Autodesk Inventor part; units mm, degrees
ref_plane "Work Plane1" through (0, 0, 7.82) normal (0, 0, 1) x (1, 0, 0)
ref_plane "Work Plane2" through (0, 0, 11.74) normal (0, 0, 1) x (1, 0, 0)
ref_plane "Work Plane3" through (0, 0, 14) normal (0, 0, 1) x (1, 0, 0)
sketch "Base" plane through (0, 0, 0) normal (0, 0, 1) x (1, 0, 0)
  line L0 (-20.125, 20.125) -> (20.125, 20.125)
  line L1 (20.125, 20.125) -> (20.125, -20.125)
  line L2 (20.125, -20.125) -> (-20.125, -20.125)
  line L3 (-20.125, -20.125) -> (-20.125, 20.125)
  line L4 (-15.74, 20.125) -> (-20.125, 15.74)
  line L5 (15.74, 20.125) -> (20.125, 15.74)
  line L6 (-17.02, 17.02) -> (17.02, 17.02) construction
  line L7 (17.02, 17.02) -> (17.02, -17.02) construction
  line L8 (17.02, -17.02) -> (-17.02, -17.02) construction
  line L9 (-17.02, -17.02) -> (-17.02, 17.02) construction
  line L10 (-17.02, 17.02) -> (17.02, -17.02) construction
  line L11 (17.02, 17.02) -> (-17.02, -17.02) construction
  circle A0 centre (0, 0) radius 8.4
  circle A1 centre (17.02, 17.02) radius 1.05
  circle A2 centre (-17.02, 17.02) radius 1.05
  circle A3 centre (-17.02, -17.02) radius 1.05
  circle A4 centre (17.02, -17.02) radius 1.05
  line L12 (-20.125, -15.74) -> (-15.74, -20.125)
  line L13 (20.125, -15.74) -> (15.74, -20.125)
  point P0 (0, 0)
  point P1 (0, 0)
  dimension "d0" = 40.25
  dimension "d1" = 40.25
  dimension "d2" = 135
  dimension "d3" = 135
  dimension "d4" = 31.48
  dimension "d5" = 34.04
  dimension "d6" = 3.105
  dimension "d7" = 3.105
  dimension "d8" = 3.105
  dimension "d9" = 3.105
  dimension "d10" = 16.8
  dimension "d11" = 2.1
  dimension "d12" = 135
  dimension "d13" = 135
  dimension "d14" = 31.48
  dimension "d15" = 34.04
  dimension "d16" = 31.48
extrude "BaseFeature" add sketch "Base" along normal blind 1.5 contours L0 L5 L1 L13 L2 L12 L3 L4 | A0
extrude "CameraFeature" add sketch "Base" along normal blind 16 contours A0
sketch "Sketch2" plane through (0, 0, 16) normal (0, 0, 1) x (1, 0, 0)
  circle A0 centre (0, 0) radius 8.4
  circle A1 centre (0, 0) radius 4
  point P0 (0, 0)
  dimension "d28" = 8
extrude "Extrusion3" cut sketch "Sketch2" against normal blind 7.62 contours A1
sketch "Sketch4" plane through (0, 0, 1.5) normal (0, 0, 1) x (1, 0, 0)
  circle A0 centre (0, 0) radius 4
  circle A1 centre (0, 0) radius 8.4
  line L0 (-8.4, -8.4) -> (8.4, -8.4)
  line L1 (8.4, -8.4) -> (8.4, 8.4)
  line L2 (8.4, 8.4) -> (-8.4, 8.4)
  line L3 (-8.4, 8.4) -> (-8.4, -8.4)
  circle A2 centre (0, 0) radius 8.4
  point P0 (0, 0)
extrude "Extrusion5" add sketch "Sketch4" along normal blind 4.32 contours A0 | A1 | L1 L0 A1 | A1 L2 L1 | A1 L3 L2 | L0 L3 A1
ref_plane "Work Plane1" through (0, 0, 7.82) normal (0, 0, 1) x (1, 0, 0)
ref_plane "Work Plane2" through (0, 0, 11.74) normal (0, 0, 1) x (1, 0, 0)
sketch "Sketch5" plane through (0, 0, 7.82) normal (0, 0, 1) x (1, 0, 0)
  circle A0 centre (0, 0) radius 8.4
  circle A1 centre (0, 0) radius 5.64
  point P0 (0, 0)
  dimension "d33" = 11.28
extrude "Extrusion6" cut sketch "Sketch5" along normal up to surface (3.92 mm away)
ref_plane "Work Plane3" through (0, 0, 14) normal (0, 0, 1) x (1, 0, 0)
sketch "Sketch6" plane through (0, 0, 16) normal (0, 0, 1) x (1, 0, 0)
  circle A0 centre (0, 0) radius 8.4
  point P0 (0, 0)
sketch "Sketch7" plane through (0, 0, 14) normal (0, 0, 1) x (1, 0, 0)
  circle A0 centre (0, 0) radius 4
  point P0 (0, 0)
loft "Loft1" cut profiles "Sketch7" section 2 edges at (-8.4, 0, 16)
sketch "Sketch8" plane through (0, 0, 1.5) normal (0, 0, 1) x (1, 0, 0)
  line L0 (8.4, 8.4) -> (0, 8.4)
  line L1 (0, 8.4) -> (-8.4, 8.4)
  line L2 (0, -8.4) -> (8.4, -8.4)
  line L3 (-8.4, -8.4) -> (0, -8.4)
  line L4 (15.74, 20.125) -> (-15.74, 20.125) construction
  line L5 (0, 20.125) -> (0, 8.4) construction
  line L6 (0, -8.4) -> (0, -20.125) construction
  line L7 (-15.74, -20.125) -> (15.74, -20.125) construction
  circle A0 centre (0, 10.4) radius 2.12
  line L8 (2.12, 10.4) -> (-2.12, 10.4) construction
  line L9 (-2.12, 10.4) -> (-2.12, 8.4)
  line L10 (-2.12, 8.4) -> (2.12, 8.4)
  line L11 (2.12, 8.4) -> (2.12, 10.4)
  line L12 (-28.175, 0) -> (28.175, 0)
  circle A1 centre (0, -10.4) radius 2.12
  line L13 (-2.12, -10.4) -> (-2.12, -8.4)
  line L14 (-2.12, -8.4) -> (2.12, -8.4)
  line L15 (2.12, -8.4) -> (2.12, -10.4)
  point P0 (0, 0)
  dimension "d41" = 4.24
  dimension "d42" = 2
extrude "Extrusion7" add sketch "Sketch8" along normal blind 4.32 contours L0 A0 L11 | L0 L1 A0 | L1 L9 A0 | L2 A1 L3 | L2 L15 A1 | A1 L13 L3 picked at (0, 11.1364) picked at (0, -11.1364)
sketch "Sketch9" plane through (0, 0, 1.5) normal (0, 0, 1) x (1, 0, 0)
  line L0 (20.06, 8.4) -> (15.7, 8.4)
  line L1 (15.7, 8.4) -> (15.7, -8.4)
  line L2 (15.7, -8.4) -> (20.06, -8.4)
  line L3 (20.06, -8.4) -> (20.06, 8.4)
  line L4 (8.4, 8.4) -> (2.12, 8.4)
  line L5 (2.12, -8.4) -> (8.4, -8.4)
  line L6 (8.4, -8.4) -> (8.4, 0)
  point P0 (0, 0)
  dimension "d45" = 4.36
  dimension "d46" = 7.3
extrude "Extrusion8" add sketch "Sketch9" along normal blind 2
equation "\"d1\" = d0"
equation "\"d3\" = d2"
equation "\"d7\" = d6"
equation "\"d9\" = d8"
equation "\"d12\" = d2"
equation "\"d13\" = d2"
equation "\"d14\" = d4"
properties part number "Arducam"
The listing builds one solid part. Answer for the finished solid, in the listing's coordinates (mm). A direction names the side the tool comes from. Round coordinates to 2 decimals unless told otherwise and drop trailing zeros. Write each loop counter-clockwise with the first axis right and the second up, starting at its lowest first coordinate (ties: lowest second). Pieces come first, ordered by that corner, then holes. Notation, with made-up numbers: (-12, 58.25) -> (-7, 58.25) arc R20 cw to (-7, 63.25) -> close; hole circle Ø10 at (22, 29). An arc over 180 degrees is marked (long way). Use CSV: the item, a comma, the result in double quotes. Start each with the question number.
(1) Which of the six approach directions +Z, -Z, +X, -X, +Y, -Y give full straight-line access (tool end or side, diameter ignored) to faces 1 (the face through (1, -9, 5.82)), 2 (the face through (8.012, -2.523, 13.84)), 3 (the face through (5.21, 2.16, 9.75)), 4 (the face through (2.12, 9, 4)), 5 (the face through (15.7, 0, 2))?
(2) Section D-D on x = 17.02 is taken. Give the vertices of the cut face in (y, z) (3 decimals).
(3) Section C-C on z = 12.75 is taken. Give the vertices of the cut face in (x, y).
(4) Section A-A on x = -17.02 is taken. Give the vertices of the cut face in (y, z) (3 decimals).
(5) The mould has two halves that part along X. Classify faces 6 (the face through (8.4, 0, 4)), 7 (the face through (-17.902, 17.963, 0.74)), 8 (the face through (-2, -5.5, 11.74)): released by +X, released by -X, zero draft, split by the parting line, or undercut.
(6) Consider L1, parallel to Y at x = -17.02, z = 1 (3 decimals); L2, parallel to X at y = 4.5, z = 2.75; L3, parallel to Y at x = 0, z = 10.4. Determine where each line is inside the solid, lowest interval first. Write a range as from..to.
(7) Each of these flat-tipped pins is pushed along its axis until it touches: pin 1 (1 mm diameter, centred on x = 18.5, z = 3, fed in from +Y); pin 2 (1.6 mm diameter, centred on y = 9, z = 3, fed in from +X); pin 3 (7 mm diameter, centred on x = 0, y = 0, fed in from +Z); pin 4 (4 mm diameter, centred on x = 4, z = 3, fed in from -Y) (3 decimals). Where does it stop, or does it pass through?
A:
1,face 1,"+Z, -Y"
1,face 2,"+Z"
1,face 3,"none"
1,face 4,"+Z, +X, +Y"
1,face 5,"+Z, +Y, -Y"
2,outline,"(-18.845, 0) -> (-18.07, 0) -> (-18.07, 1.5) -> (-18.845, 1.5) -> close; (-15.97, 0) -> (15.97, 0) -> (15.97, 1.5) -> (8.4, 1.5) -> (8.4, 3.5) -> (-8.4, 3.5) -> (-8.4, 1.5) -> (-15.97, 1.5) -> close; (18.07, 0) -> (18.845, 0) -> (18.845, 1.5) -> (18.07, 1.5) -> close"
3,outline,"circle Ø16.8 at (0, 0); hole circle Ø8 at (0, 0)"
4,outline,"(-18.845, 0) -> (-18.07, 0) -> (-18.07, 1.5) -> (-18.845, 1.5) -> close; (-15.97, 0) -> (15.97, 0) -> (15.97, 1.5) -> (-15.97, 1.5) -> close; (18.07, 0) -> (18.845, 0) -> (18.845, 1.5) -> (18.07, 1.5) -> close"
5,face 6,"undercut"
5,face 7,"released by -X"
5,face 8,"zero draft"
6,L1,"y = -18.845..-18.07, -15.97..15.97, 18.07..18.845"
6,L2,"x = -8.4..8.4, 15.7..20.06"
6,L3,"y = -5.64..-4, 4..5.64"
7,pin 1,"stops at y = 8.4"
7,pin 2,"stops at x = 20.06"
7,pin 3,"stops at z = 8.38"
7,pin 4,"stops at y = -20.125"
